```python
from build123d import *

# Parameters (mm, degrees)
F2_DEPTH = 12.7
F3_R     = 19.05
F4_DEPTH = 12.7
F5_DEPTH = 12.7


# Not quite as in the source:
# - a variable given as a bare number and used for a length is read in inches; the dataset says mm whatever the document's units were


with BuildPart() as f2:
    # F1 (on Top) → F2 (new body)
    with BuildSketch(Plane.XY):
        with BuildLine():
            Line((-76.2, -25.4), (76.2, -25.4))
            ThreePointArc((76.2, -25.4), (101.6, 0), (76.2, 25.4))
            Line((76.2, 25.4), (-76.2, 25.4))
            ThreePointArc((-76.2, 25.4), (-101.6, 0), (-76.2, -25.4))
        make_face()
    extrude(amount=F2_DEPTH)

    # F3 (on face) → F4 (join)
    with BuildSketch(Plane.XY.offset(12.7)):
        with Locations((-76.2, 0)):
            Circle(F3_R)
    extrude(amount=F4_DEPTH)

    # F3 (on face) → F5 (cut)
    with BuildSketch(Plane.XY.offset(12.7)):
        with Locations((76.2, 0)):
            Circle(F3_R)
    extrude(amount=-F5_DEPTH, mode=Mode.SUBTRACT)


solid = f2.part
```
Model file for the job. Use its own axes, mm. Coordinates: 2 decimals unless noted, no trailing zeros. Loops run counter-clockwise (first coordinate to the right, second up) from the corner with the lowest first, then second, coordinate; pieces in that order, holes last. Notation, with made-up numbers: (-0.75, 62.25) - (39.25, 62.25) arc R11 ccw to (39.25, 75.25) - close; hole circle Ø4 at (-17, 39). An arc over 180 degrees is marked (long way). Write item = value, one per line. Start each with the question number.
Item 1: Saw through at B-B, the plane y = 11. List the corners of the cut face in (x, z).
Item 2: Saw through at A-A, the plane y = 0. List the corners of the cut face in (x, z), then the cut area to 3 significant figures.
Item 3: Saw through at D-D, the plane z = 22.75. List the corners of the cut face in (x, y).
Item 4: Pull direction X, two halves, no side cores. Call faces 1 (the face through (-58.03, 5.72, 18.96)), 2 (the face through (-24, 0, 0)), 3 (the face through (57.17, 0.84, 6.44)), 4 (the face through (-101.594, 0.559, 6.261)): +X half, -X half, draft (parallel to the pull), parting line (faces both ways), or undercut.
Item 5: Drop flat-ended pins along their axis: pin 1 Ø1 at (y, z) = (-12, 9.5) entering from -X; pin 2 Ø10 at (x, y) = (23, -11.5) entering from +Z; pin 3 Ø4 at (y, z) = (-0.5, 19) entering from +X. Give the stop position or say it passes through.
Item 6: Saw through at C-C, the plane x = 37.5. List the corners of the cut face in (y, z).
Item 7: Wall check: probe 1 along Y at (x, z) = (76.2, 3.75); probe 2 along Z at (x, y) = (34, -12.5); probe 3 along Y at (x, z) = (62.5, 6.75). Give the ranges that are in metal, low to high. Write a range as [from, to].
Answers:
q1.outline = (-99.09, 0) - (60.65, 0) - (60.65, 12.7) - (-60.65, 12.7) - (-60.65, 25.4) - (-91.75, 25.4) - (-91.75, 12.7) - (-99.09, 12.7) - close; (91.75, 0) - (99.09, 0) - (99.09, 12.7) - (91.75, 12.7) - close
q2.outline = (-101.6, 0) - (57.15, 0) - (57.15, 12.7) - (-57.15, 12.7) - (-57.15, 25.4) - (-95.25, 25.4) - (-95.25, 12.7) - (-101.6, 12.7) - close; (95.25, 0) - (101.6, 0) - (101.6, 12.7) - (95.25, 12.7) - close
q2.area = 2,580 mm2
q3.outline = circle Ø38.1 at (-76.2, 0)
q4.face_1 = parting line
q4.face_2 = draft
q4.face_3 = undercut
q4.face_4 = -X half
q5.pin_1 = -98.85
q5.pin_2 = 12.7
q5.pin_3 = -57.15
q6.outline = (-25.4, 0) - (25.4, 0) - (25.4, 12.7) - (-25.4, 12.7) - close
q7.probe_1 = [-25.4, -19.05], [19.05, 25.4]
q7.probe_2 = [0, 12.7]
q7.probe_3 = [-25.4, -13.24], [13.24, 25.4]
